Could you check a few things on this model? Use its own coordinates, in mm. Face numbers are marked on the shaded views. Give positions to 0.01 mm unless a question says otherwise; leave off trailing zeros. Order: outer loops, then holes, each group sorted by start corner. A loop starts at its lowest first (then second) coordinate and runs counter-clockwise, first axis right, second up. Notation, with made-up numbers: (77, 13) -> (92, 13) arc R26 cw to (92, 27) -> close; hole circle Ø7 at (89.5, 33.5). An arc over 180 degrees is marked (long way). Write each question's results on one line, items separated by ' | '.
```python
from build123d import *

# Parameters (mm, degrees)
PAD010_DEPTH    = 2
PAD011_DEPTH    = 5.4
SKETCH023_W     = 40
SKETCH023_H     = 30
SKETCH023_W_2   = 2.5
SKETCH023_H_2   = 95.99
SKETCH023_W_3   = 113.7
SKETCH023_H_3   = 2.5
SKETCH023_W_4   = 22.3
SKETCH023_W_5   = 46.56
SKETCH023_W_6   = 2.45
SKETCH023_H_4   = 75.89
PAD012_DEPTH    = 9.4
POCKET_DEPTH    = 26
SKETCH025_W     = 15
SKETCH025_H     = 10
POCKET008_DEPTH = 6
SKETCH028_W     = 22.31
SKETCH028_H     = 1.8
PAD015_DEPTH    = 10.4
FILLET_R        = 5
FILLET001_R     = 3
SKETCH035_W     = 6
SKETCH035_H     = 1.5
POCKET011_DEPTH = 1.2
SKETCH036_W     = 6
SKETCH036_H     = 1.5
POCKET012_DEPTH = 1.2
SKETCH037_R     = 1.1
POCKET013_DEPTH = 12
SKETCH038_R     = 2
POCKET014_DEPTH = 5
SKETCH051_W     = 2.45
SKETCH051_H     = 4
POCKET023_DEPTH = 4
SKETCH055_W     = 2.45
SKETCH055_H     = 5.4
POCKET024_DEPTH = 12.87


with BuildPart() as part:
    # Sketch020 → Pad010 (new body)
    with BuildSketch(Plane.XY):
        with BuildLine():
            Line((235.7, -27.1), (235.7, -125.39))
            ThreePointArc((231.7, -129.39), (234.528427, -128.218427), (235.7, -125.39))
            Line((156.44, -129.39), (231.7, -129.39))
            Line((156.44, -129.39), (156.44, -137.19))
            Line((116.44, -137.19), (156.44, -137.19))
            Line((116.44, -129.39), (116.44, -137.19))
            Line((116.44, -129.39), (90.44, -129.39))
            ThreePointArc((86.44, -125.39), (87.611573, -128.218427), (90.44, -129.39))
            Line((86.44, -27.1), (86.44, -125.39))
            ThreePointArc((90.44, -23.1), (87.611573, -24.271573), (86.44, -27.1))
            Line((90.44, -23.1), (231.7, -23.1))
            ThreePointArc((235.7, -27.1), (234.528427, -24.271573), (231.7, -23.1))
        make_face()
    extrude(amount=PAD010_DEPTH)

    # Sketch021 (on Face14 of Pad010) → Pad011 (join)
    with BuildSketch(Plane.XY.offset(2)):
        with BuildLine():
            Line((235.7, -27.1), (235.7, -125.39))
            ThreePointArc((231.7, -129.39), (234.528427, -128.218427), (235.7, -125.39))
            Line((231.7, -129.39), (181.44, -129.39))
            Line((181.44, -127.59), (181.44, -129.39))
            Line((228, -127.59), (181.44, -127.59))
            Line((228, -127.59), (228, -124.99))
            ThreePointArc((229, -123.99), (228.292893, -124.282893), (228, -124.99))
            Line((233.9, -123.99), (229, -123.99))
            Line((233.9, -123.99), (233.9, -24.9))
            Line((230.15, -24.9), (233.9, -24.9))
            Line((230.15, -24.9), (230.15, -23.1))
            Line((230.15, -23.1), (231.7, -23.1))
            ThreePointArc((235.7, -27.1), (234.528427, -24.271573), (231.7, -23.1))
        make_face()
        with BuildLine():
            Line((86.44, -27.1), (86.44, -125.39))
            ThreePointArc((86.44, -125.39), (87.611573, -128.218427), (90.44, -129.39))
            Line((90.44, -129.39), (116.44, -129.39))
            Line((116.44, -129.39), (116.44, -127.59))
            Line((116.44, -127.59), (94.14, -127.59))
            Line((94.14, -124.99), (94.14, -127.59))
            ThreePointArc((94.14, -124.99), (93.847107, -124.282893), (93.14, -123.99))
            Line((88.24, -123.99), (93.14, -123.99))
            Line((88.24, -28), (88.24, -123.99))
            Line((93.14, -28), (88.24, -28))
            ThreePointArc((93.14, -28), (93.847107, -27.707107), (94.14, -27))
            Line((94.14, -24.9), (94.14, -27))
            Line((207.84, -24.9), (94.14, -24.9))
            Line((207.84, -24.9), (207.84, -23.1))
            Line((90.44, -23.1), (207.84, -23.1))
            ThreePointArc((90.44, -23.1), (87.611573, -24.271573), (86.44, -27.1))
        make_face()
    extrude(amount=PAD011_DEPTH)

    # Sketch023 (on Face3 of Pad011) → Pad012 (join)
    with BuildSketch(Plane.XY.offset(2)):
        with Locations((136.44, -122.19)):
            Rectangle(SKETCH023_W, SKETCH023_H)
        with Locations((89.49, -75.995)):
            Rectangle(SKETCH023_W_2, SKETCH023_H_2)
        with Locations((150.99, -26.15)):
            Rectangle(SKETCH023_W_3, SKETCH023_H_3)
        with Locations((105.29, -126.34)):
            Rectangle(SKETCH023_W_4, SKETCH023_H_3)
        with Locations((204.72, -126.34)):
            Rectangle(SKETCH023_W_5, SKETCH023_H_3)
        with Locations((232.675, -86.045)):
            Rectangle(SKETCH023_W_6, SKETCH023_H_4)
    extrude(amount=PAD012_DEPTH)

    # Sketch024 (on Face48 of Pad012) → Pocket (cut)
    with BuildSketch(Plane.YZ.offset(156.44)):
        Polygon((-131.94, 5.4), (-131.94, 2), (-112.44, 2), (-112.44, 5.4), (-110.69, 5.4), (-110.69, 7.9), (-112.44, 7.9), (-112.44, 11.4), (-131.94, 11.4), (-131.94, 7.9), (-133.69, 7.9), (-133.69, 5.4), align=None)
    extrude(amount=-POCKET_DEPTH, mode=Mode.SUBTRACT)

    # Sketch025 (on Face61 of Pocket) → Pocket008 (cut)
    with BuildSketch(Plane.XY.offset(11.4)):
        with Locations((232.43, -51.97)):
            Rectangle(SKETCH025_W, SKETCH025_H)
    extrude(amount=-POCKET008_DEPTH, mode=Mode.SUBTRACT)

    # Sketch028 (on Face16 of Pocket008) → Pad015 (join)
    with BuildSketch(Plane.XY.offset(2)):
        with Locations((218.995, -24)):
            Rectangle(SKETCH028_W, SKETCH028_H)
    extrude(amount=PAD015_DEPTH)

    # Fillet
    fillet_edges = [part.edges().sort_by_distance(p)[0] for p in [
        (116.44, -137.19, 5.7),
        (116.44, -107.19, 6.7),
    ]]
    fillet(fillet_edges, radius=FILLET_R)

    # Fillet001
    fillet001_edges = [part.edges().sort_by_distance(p)[0] for p in [
        (156.44, -137.19, 5.7),
        (156.44, -107.19, 6.7),
    ]]
    fillet(fillet001_edges, radius=FILLET001_R)

    # Sketch035 (on Face12 of Fillet001) → Pocket011 (cut)
    with BuildSketch(Plane(origin=(88.24, 0, 0), x_dir=(0, -1, 0), z_dir=(-1, 0, 0))):
        with Locations((32.1, 8.15)):
            Rectangle(SKETCH035_W, SKETCH035_H)
        with Locations((120.39, 8.15)):
            Rectangle(SKETCH035_W, SKETCH035_H)
    extrude(amount=-POCKET011_DEPTH, mode=Mode.SUBTRACT)

    # Sketch036 (on Face68 of Pocket011) → Pocket012 (cut)
    with BuildSketch(Plane.YZ.offset(233.9)):
        with Locations((-120.39, 8.15)):
            Rectangle(SKETCH036_W, SKETCH036_H)
        with Locations((-65.97, 8.15)):
            Rectangle(SKETCH036_W, SKETCH036_H)
    extrude(amount=-POCKET012_DEPTH, mode=Mode.SUBTRACT)

    # Sketch037 (on Face16 of Pocket012) → Pocket013 (cut)
    with BuildSketch(Plane.XY.offset(11.4)):
        with Locations((124.44, -111.69)):
            Circle(SKETCH037_R)
        with Locations((124.44, -132.69)):
            Circle(SKETCH037_R)
    extrude(amount=-POCKET013_DEPTH, mode=Mode.SUBTRACT)

    # Sketch038 (on Face1 of Pocket013) → Pocket014 (cut)
    with BuildSketch(Plane(origin=(0, 0, 0), x_dir=(1, 0, 0), z_dir=(0, 0, -1))):
        with Locations((124.44, 132.69)):
            Circle(SKETCH038_R)
        with Locations((124.44, 111.69)):
            Circle(SKETCH038_R)
    extrude(amount=-POCKET014_DEPTH, mode=Mode.SUBTRACT)

    # Sketch051 (on Face29 of Pocket014) → Pocket023 (cut)
    with BuildSketch(Plane(origin=(0, -56.97, 0), x_dir=(-1, 0, 0), z_dir=(0, 1, 0))):
        with Locations((-232.675, 9.4)):
            Rectangle(SKETCH051_W, SKETCH051_H)
    extrude(amount=-POCKET023_DEPTH, mode=Mode.SUBTRACT)

    # Sketch055 (on Face72 of Pocket023) → Pocket024 (cut)
    with BuildSketch(Plane(origin=(0, -48.1, 0), x_dir=(-1, 0, 0), z_dir=(0, 1, 0))):
        with Locations((-232.675, 4.7)):
            Rectangle(SKETCH055_W, SKETCH055_H)
    extrude(amount=-POCKET024_DEPTH, mode=Mode.SUBTRACT)


solid = part.part
```
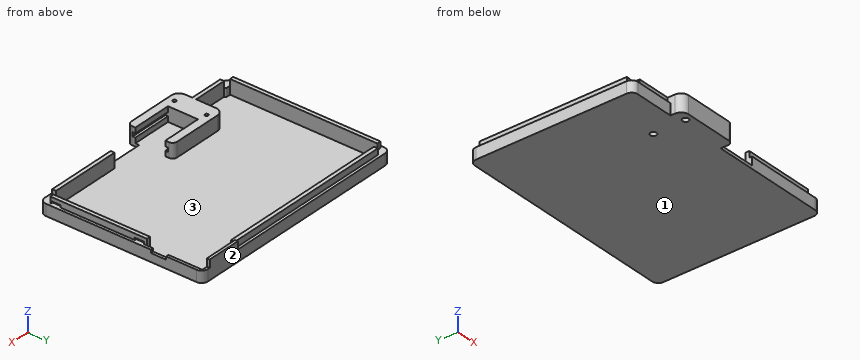
Q1. Suppose I cut it at C-C on y = -65. Please give me the cut outline in (x, z), and give its area (3 significant figures).
Here are the results:
outline: (86.44, 0) -> (235.7, 0) -> (235.7, 7.4) -> (232.7, 7.4) -> (232.7, 8.9) -> (233.9, 8.9) -> (233.9, 11.4) -> (231.45, 11.4) -> (231.45, 2) -> (90.74, 2) -> (90.74, 11.4) -> (88.24, 11.4) -> (88.24, 7.4) -> (86.44, 7.4) -> close | area: 363 mm²
Q2. Suppose I cut it at A-A on y = -53. Please give me the cut outline in (x, z), and give its area (3 significant figures).
Here are the results:
outline: (86.44, 0) -> (235.7, 0) -> (235.7, 5.4) -> (233.9, 5.4) -> (233.9, 2) -> (90.74, 2) -> (90.74, 11.4) -> (88.24, 11.4) -> (88.24, 7.4) -> (86.44, 7.4) -> close | area: 338 mm²
Q3. Thinking about a two-plate mould opening in Y: for the marked faces 1, 2 and 3, which applies, +Y half, -Y half, draft (parallel to the pull), parting line (faces both ways), or undercut?
Here are the results:
face 1: draft | face 2: +Y half | face 3: undercut
Q4. Suppose I cut it at D-D on x = 167.5. Please give me the cut outline in (y, z).
Here are the results:
outline: (-129.39, 0) -> (-23.1, 0) -> (-23.1, 7.4) -> (-24.9, 7.4) -> (-24.9, 11.4) -> (-27.4, 11.4) -> (-27.4, 2) -> (-129.39, 2) -> close
Q5. I need wall thicknesses on line 1 along Y through (x, z) = (124.44, 3.9); line 2 along X through (y, z) = (-111.69, 2.2); line 3 along X through (y, z) = (-111.69, 7.5). Which ranges of each line are inside material? Lowest first, please.
Here are the results:
line 1: y = -137.19 to -134.69, -130.69 to -113.69, -109.69 to -107.19, -27.4 to -23.1 | line 2: x = 86.44 to 90.74, 116.47 to 122.44, 126.44 to 156.44, 231.45 to 235.7 | line 3: x = 88.24 to 90.74, 116.47 to 123.34, 125.54 to 130.44, 231.45 to 233.9
Q6. Suppose I cut it at B-B on x = 150. Please give me the cut outline in (y, z).
Here are the results:
outline: (-137.19, 0) -> (-23.1, 0) -> (-23.1, 7.4) -> (-24.9, 7.4) -> (-24.9, 11.4) -> (-27.4, 11.4) -> (-27.4, 2) -> (-107.19, 2) -> (-107.19, 11.4) -> (-112.44, 11.4) -> (-112.44, 7.9) -> (-110.69, 7.9) -> (-110.69, 5.4) -> (-112.44, 5.4) -> (-112.44, 2) -> (-131.94, 2) -> (-131.94, 5.4) -> (-133.69, 5.4) -> (-133.69, 7.9) -> (-131.94, 7.9) -> (-131.94, 11.4) -> (-137.19, 11.4) -> close
Q7. I'm going to push flat-ended pins straight in: pin 1 Ø2 at (x, z) = (234.5, 6.5) entering from -Y; pin 2 Ø0.9 at (x, y) = (234.5, -50.5) entering from +Z; pin 3 Ø6 at (x, z) = (190.5, 10) entering from -Y. Where does each tip first touch, or does it pass through?
Here are the results:
pin 1: stops at y = -128.96 | pin 2: stops at z = 5.4 | pin 3: stops at y = -129.39
